Solid Edge part; units mm, degrees
sketch "Sketch1" plane through (0, 0, 0) normal (0, 0, 1) x (1, 0, 0)
  circle A0 centre (0, 0) radius 3.3
extrude "Protrusion1" add sketch "Sketch1" along normal blind 3.8
sketch "Sketch2" plane through (0, 0, 3.8) normal (0, 0, 1) x (1, 0, 0)
  circle A0 centre (0, 0) radius 2.25
extrude "Extrusionsausschnitt_1" cut sketch "Sketch2" against normal blind 1
sketch "Sketch3" plane through (0, 0, 0) normal (0, 0, -1) x (1, 0, 0)
  circle A0 centre (0, 0) radius 2.3
extrude "Extrusionsausschnitt_2" cut sketch "Sketch3" against normal blind 2
sketch "Sketch4" plane through (0, 0, 2.8) normal (0, 0, 1) x (0, 1, 0)
  circle A0 centre (0, 0) radius 1.2
extrude "Cutout1" cut sketch "Sketch4" against normal through all
sketch "Sketch5" plane through (0, 0, 3.8) normal (0, 0, 1) x (0, 1, 0)
  line L0 (-14.5, 1.8) -> (-2.1541, 2.5)
  arc A0 (-2.1541, 2.5) -> (-2.1541, -2.5) centre (0, 0) ccw
  line L1 (-14.5, -1.8) -> (-2.1541, -2.5)
  arc A1 (-14.5, 1.8) -> (-14.5, -1.8) centre (-14.17, 0) ccw
  line L2 (2.1541, 2.5) -> (14.5, 1.8)
  arc A2 (14.5, 1.8) -> (14.5, -1.8) centre (14.17, 0) cw
  line L3 (2.1541, -2.5) -> (14.5, -1.8)
  arc A3 (2.1541, 2.5) -> (2.1541, -2.5) centre (0, 0) cw
  dimension "D1" = 14.5
  dimension "D2" = 2.1541
  dimension "D3" = 2.1541
  dimension "D4" = 2.1541
  dimension "D5" = 2.1541
  dimension "D6" = 14.5
  dimension "D7" = 14.5
extrude "Extrusionsausprägung_2" add sketch "Sketch5" against normal blind 1.4
sketch "Sketch6" plane through (0, 0, 0) normal (0, 0, 1) x (1, 0, 0)
  circle A0 centre (0, -14.15) radius 0.6
  circle A1 centre (0, -12.25) radius 0.6
  circle A2 centre (0, -10.35) radius 0.6
  circle A3 centre (0, -8.45) radius 0.6
  circle A4 centre (0, -6.55) radius 0.6
  circle A5 centre (0, -4.65) radius 0.6
extrude "Cutout2" cut sketch "Sketch6" along normal through all
mirror "Mirror1" about plane through (0, 0, 0) normal (0, -1, 0) of "Cutout2"
CAD build for the part. Positions are in the model's coordinates, mm. A direction names the side the tool comes from. Round coordinates to 2 decimals unless told otherwise and drop trailing zeros. Write each loop counter-clockwise with the first axis right and the second up, starting at its lowest first coordinate (ties: lowest second). Pieces come first, ordered by that corner, then holes. Notation, with made-up numbers: (56.5, 8.25) -> (107.5, 8.25) arc R21 ccw to (107.5, 21.25) -> close; hole circle Ø10 at (-1.5, 67). An arc over 180 degrees is marked (long way). Answer in a Markdown table with one row per item. Add a question column.
Item 1: Saw through at D-D, the plane x = 3. Write the cut outline in (y, z).
Item 2: Which spindle directions (+Z, -Z, +X, -X, +Y, -Y) get a long thin tool onto all of the face, cutting with end or side? Do faces 4 (the face through (2.145, -8.413, 3.11)), 5 (the face through (-1, -1, 2)), 6 (the face through (-0.29, 2.23, 3.31)). Say none if no direction does.
Item 3: Saw through at B-B, the plane z = 3.3. Count the separate pieces of the cut face and the enclosed holes in it, then the cut area to 3 significant figures.
Item 4: Mould opens along X. For faces 1 (the face through (1, -1, 2.8)), 2 (the face through (-2.145, -8.413, 3.11)), 3 (the face through (1.4, -2.2, 0)) say: pulls with the +X half, pulls with the -X half, needs draft (parallel to the pull), parting line crosses it, or undercut.
Item 5: Drill centre lines: line 1 (X direction, y = 0, z = 0.35); line 2 (X direction, y = 0, z = 2.3); line 3 (Z direction, x = -2, y = 6). Where is each one in solid material? Low to high. Write a range as from..to.
Item 6: Saw through at A-A, the plane y = 0. Write the cut outline in (x, z), then the cut area to 3 significant figures.
Item 7: Saw through at C-C, the plane y = -10.35. Write the cut outline in (x, z), then the cut area to 3 significant figures.
Item 8: Drop flat-ended pins along their axis: pin 1 Ø1.5 at (x, y) = (-1, 7.5) entering from -Z; pin 2 Ø1.1 at (x, y) = (0, 6.55) entering from -Z (3 decimals); pin 3 Ø3 at (x, y) = (0, 0) entering from +Z; pin 4 Ø3.5 at (x, y) = (0, 0) entering from -Z. Give the stop position or say it passes through.
Findings below:
| question | item | result |
|---|---|---|
| 1 | outline | (-1.37, 0) -> (1.37, 0) -> (1.37, 3.8) -> (-1.37, 3.8) -> close |
| 2 | face 4 | +Z, -Z, +X, -Y |
| 2 | face 5 | -Z |
| 2 | face 6 | +Z |
| 3 | separate pieces | 1 |
| 3 | enclosed holes | 13 |
| 3 | area | 111 mm^2 |
| 4 | face 1 | undercut |
| 4 | face 2 | pulls with the -X half |
| 4 | face 3 | needs draft |
| 5 | line 1 | x = -3.3..-2.3, 2.3..3.3 |
| 5 | line 2 | x = -3.3..-1.2, 1.2..3.3 |
| 5 | line 3 | z = 2.4..3.8 |
| 6 | outline | (-3.3, 0) -> (-2.3, 0) -> (-2.3, 2) -> (-1.2, 2) -> (-1.2, 2.8) -> (-2.25, 2.8) -> (-2.25, 3.8) -> (-3.3, 3.8) -> close; (1.2, 2) -> (2.3, 2) -> (2.3, 0) -> (3.3, 0) -> (3.3, 3.8) -> (2.25, 3.8) -> (2.25, 2.8) -> (1.2, 2.8) -> close |
| 6 | area | 9.46 mm^2 |
| 7 | outline | (-2.04, 2.4) -> (-0.6, 2.4) -> (-0.6, 3.8) -> (-2.04, 3.8) -> close; (0.6, 2.4) -> (2.04, 2.4) -> (2.04, 3.8) -> (0.6, 3.8) -> close |
| 7 | area | 4.02 mm^2 |
| 8 | pin 1 | stops at z = 2.4 |
| 8 | pin 2 | passes through |
| 8 | pin 3 | stops at z = 2.8 |
| 8 | pin 4 | stops at z = 2 |
